from build123d import *

# Parameters (mm, degrees)
SKETCH1_R           = 5
BOSS_EXTRUDE1_DEPTH = 6.25
SKETCH2_R           = 3
BOSS_EXTRUDE2_DEPTH = 20
SKETCH3_R           = 2.25
BOSS_EXTRUDE3_DEPTH = 50
SKETCH4_R           = 2.5
CUT_EXTRUDE1_DEPTH  = 40
CUT_EXTRUDE2_START  = -12.5
SKETCH5_R           = 3.75
CUT_EXTRUDE2_DEPTH  = 10


with BuildPart() as part:
    # Sketch1 → Boss-Extrude1 (new body, symmetric)
    with BuildSketch(Plane.XY):
        Circle(SKETCH1_R)
    extrude(amount=BOSS_EXTRUDE1_DEPTH, both=True)

    # Sketch2 → Boss-Extrude2 (add, symmetric)
    with BuildSketch(Plane(origin=(0, 0, 0), x_dir=(1, 0, 0), z_dir=(0, 1, 0))):
        with Locations((0, -1.25)):
            Circle(SKETCH2_R)
    extrude(amount=BOSS_EXTRUDE2_DEPTH, both=True)

    # Sketch3 → Boss-Extrude3 (add)
    with BuildSketch(Plane(origin=(0, 0, 0), x_dir=(0, 0, -1), z_dir=(1, 0, 0))):
        Circle(SKETCH3_R)
    extrude(amount=BOSS_EXTRUDE3_DEPTH)

    # Sketch4 → Cut-Extrude1 (cut)
    with BuildSketch(Plane.XZ.offset(20)):
        with Locations((0, 1.25)):
            Circle(SKETCH4_R)
    extrude(amount=-CUT_EXTRUDE1_DEPTH, mode=Mode.SUBTRACT)

    # Sketch5 → Cut-Extrude2 (cut)
    with BuildSketch(Plane.XY.offset(6.25).offset(CUT_EXTRUDE2_START)):
        Circle(SKETCH5_R)
    extrude(amount=CUT_EXTRUDE2_DEPTH, mode=Mode.SUBTRACT)


solid = part.part
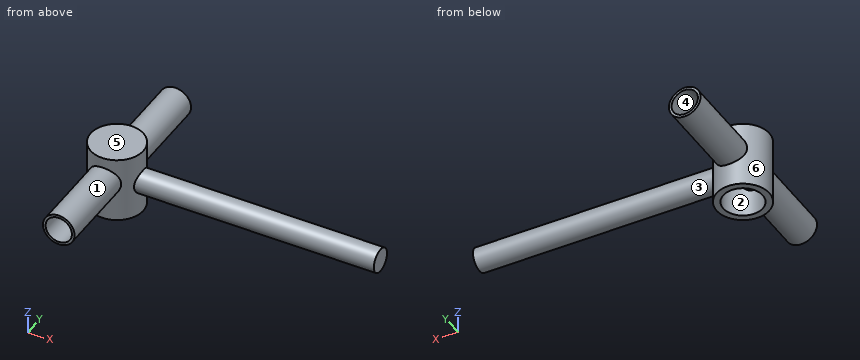
The listing builds one solid part. Answer for the finished solid, in the listing's coordinates (mm). Face numbers are marked on the shaded views. A direction names the side the tool comes from. Coordinates: 2 decimals unless noted, no trailing zeros. Loops run counter-clockwise (first coordinate to the right, second up) from the corner with the lowest first, then second, coordinate; pieces in that order, holes last. Notation, with made-up numbers: M 27,15 L 80,15 A29 cw 80,53 Z; hole C 79,-6 d10. An arc over 180 degrees is marked long. Answer in a Markdown table with one row per item.
1) Find section A-A (z = 1.25). Determine the outline of the cut face in (x, y), then the cut area to 3 significant figures.
Answers below:
| item | result |
|---|---|
| outline | M -3,-20 L -2.5,-20 L -2.5,-2.8 A3.75 cw -2.5,2.8 L -2.5,20 L -3,20 L -3,4 A5 ccw -3,-4 Z; M 2.5,-20 L 3,-20 L 3,-4 A5 ccw 4.64,-1.87 L 50,-1.87 L 50,1.87 L 4.64,1.87 A5 ccw 3,4 L 3,20 L 2.5,20 L 2.5,2.8 A3.75 cw 2.5,-2.8 Z |
| area | 222 mm^2 |
2) Given pin 1 (5 mm diameter, centred on x = 3, z = 2.5, fed in from -Y); pin 2 (1 mm diameter, centred on y = -10.5, z = -1, fed in from -X); pin 3 (12 mm diameter, centred on x = 40, y = 1.5, fed in from +Z); pin 4 (12 mm diameter, centred on x = 4, y = 12.5, fed in from -Z), each flat-ended and moving along its own axis, determine where each tip first touches the part or whether it passes through.
Answers below:
| item | result |
|---|---|
| pin 1 | y = -20 |
| pin 2 | x = -2.44 |
| pin 3 | z = 2.25 |
| pin 4 | z = -1.75 |
3) Find section D-D (y = 8.5). Determine the outline of the cut face in (x, z), then the cut area to 3 significant figures.
Answers below:
| item | result |
|---|---|
| outline | C 0,1.25 d6; hole C 0,1.25 d5 |
| area | 8.64 mm^2 |
4) Find section B-B (y = 0). Determine the outline of the cut face in (x, z), then the cut area to 4 significant figures.
Answers below:
| item | result |
|---|---|
| outline | M -5,-6.25 L -3.75,-6.25 L -3.75,3.75 L 3.75,3.75 L 3.75,-6.25 L 5,-6.25 L 5,-2.25 L 50,-2.25 L 50,2.25 L 5,2.25 L 5,6.25 L -5,6.25 Z |
| area | 252.5 mm^2 |
5) Find the intervals of material crossed by probe 1 along Z at (x, y) = (0, -6); probe 2 along X at (y, z) = (8.75, 1.25); probe 3 along Y at (x, z) = (3, -1), in increasing order.
Answers below:
| item | result |
|---|---|
| probe 1 | -1.75 to -1.25, 3.75 to 4.25 |
| probe 2 | -3 to -2.5, 2.5 to 3 |
| probe 3 | -4 to -2.25, 2.25 to 4 |
6) Find section C-C (x = 1). Determine the outline of the cut face in (y, z).
Answers below:
| item | result |
|---|---|
| outline | M -20,-1.58 L -4.9,-1.58 L -4.9,-6.25 L -3.61,-6.25 L -3.61,-1.04 L -20,-1.04 Z; M -20,3.54 L -3.61,3.54 L -3.61,3.75 L 3.61,3.75 L 3.61,3.54 L 20,3.54 L 20,4.08 L 4.9,4.08 L 4.9,6.25 L -4.9,6.25 L -4.9,4.08 L -20,4.08 Z; M 3.61,-6.25 L 4.9,-6.25 L 4.9,-1.58 L 20,-1.58 L 20,-1.04 L 3.61,-1.04 Z |
7) Which of the six approach directions +Z, -Z, +X, -X, +Y, -Y give full straight-line access (tool end or side, diameter ignored) to the marked faces 1, 2 and 3?
Answers below:
| item | result |
|---|---|
| face 1 | -Y |
| face 2 | -Z |
| face 3 | +X |
8) Determine the mould class of the marked faces 4, 5 and 6 for opening direction X: released by +X, released by -X, zero draft, split by the parting line, or undercut.
Answers below:
| item | result |
|---|---|
| face 4 | undercut |
| face 5 | zero draft |
| face 6 | split by the parting line |
